from build123d import *

# Parameters (mm, degrees)
SKETCH1_R                = 6.5
SKETCH1_R_2              = 2
BOSS_EXTRUDE1_DEPTH      = 15
BOSS_EXTRUDE2_START      = -15
BOSS_EXTRUDE2_DEPTH      = 15
FILLET1_R                = 0.6
CIRPATTERN1_COUNT        = 10
FILLET1_OF_CIRPATTERN1_R = 0.6
BOSS_EXTRUDE3_START      = -15
BOSS_EXTRUDE3_DEPTH      = 15
BOSS_EXTRUDE4_DEPTH      = 7


with BuildPart() as part:
    # Sketch1 → Boss-Extrude1 (new body)
    with BuildSketch(Plane(origin=(0, 0, 0), x_dir=(1, 0, 0), z_dir=(0, 1, 0))):
        with Locations(Location((0, 0, 0), (0, 0, 270))):
            Circle(SKETCH1_R)
        with Locations(Location((0, 0, 0), (0, 0, 270))):
            Circle(SKETCH1_R_2, mode=Mode.SUBTRACT)
    extrude(amount=BOSS_EXTRUDE1_DEPTH)

    # Sketch2 → Boss-Extrude2 (add)
    with BuildSketch(Plane(origin=(0, 15, 0), x_dir=(1, 0, 0), z_dir=(0, 1, 0)).offset(BOSS_EXTRUDE2_START)):
        with BuildLine():
            Line((0.975354337, 8.443854802), (1.342832983, 6.359779837))
            ThreePointArc((1.342832983, 6.359779837), (0, 6.5), (-1.342832983, 6.359779837))
            Line((-1.342832983, 6.359779837), (-0.975354337, 8.443854802))
            ThreePointArc((-0.975354337, 8.443854802), (0, 8.5), (0.975354337, 8.443854802))
        make_face()
    boss_extrude2 = extrude(amount=BOSS_EXTRUDE2_DEPTH)

    # Fillet1
    fillet1_edges = [part.edges().sort_by_distance(p)[0] for p in [
        (-0.975354337, 7.5, -8.443854802),
        (0.975354337, 7.5, -8.443854802),
        (1.342832983, 7.5, -6.359779837),
        (-1.342832983, 7.5, -6.359779837),
    ]]
    fillet(fillet1_edges, radius=FILLET1_R)

    # CirPattern1: Boss-Extrude2 ×10 about axis
    cirpattern1_axis = Axis((0, 0, 0), (0, 1, 0))
    for i in range(1, CIRPATTERN1_COUNT):
        add(boss_extrude2.rotate(cirpattern1_axis, i * 360 / CIRPATTERN1_COUNT))

    # Fillet1 of CirPattern1
    fillet1_of_cirpattern1_edges = [part.edges().sort_by_distance(p)[0] for p in [
        (-5.752251559, 7.5, -6.257923138),
        (-4.174095091, 7.5, -7.404520928),
        (-2.651810092, 7.5, -5.934467393),
        (-4.8245595, 7.5, -4.355872545),
        (-8.331984198, 7.5, -1.681677534),
        (-7.729182066, 7.5, -3.53691173),
        (-5.633551844, 7.5, -3.242390109),
        (-6.463468269, 7.5, -0.688169991),
        (-7.729182066, 7.5, 3.53691173),
        (-8.331984198, 7.5, 1.681677534),
        (-6.463468269, 7.5, 0.688169991),
        (-5.633551844, 7.5, 3.242390109),
        (-4.174095091, 7.5, 7.404520928),
        (-5.752251559, 7.5, 6.257923138),
        (-4.8245595, 7.5, 4.355872545),
        (-2.651810092, 7.5, 5.934467393),
        (0.975354337, 7.5, 8.443854802),
        (-0.975354337, 7.5, 8.443854802),
        (-1.342832983, 7.5, 6.359779837),
        (1.342832983, 7.5, 6.359779837),
        (5.752251559, 7.5, 6.257923138),
        (4.174095091, 7.5, 7.404520928),
        (2.651810092, 7.5, 5.934467393),
        (4.8245595, 7.5, 4.355872545),
        (8.331984198, 7.5, 1.681677534),
        (7.729182066, 7.5, 3.53691173),
        (5.633551844, 7.5, 3.242390109),
        (6.463468269, 7.5, 0.688169991),
        (7.729182066, 7.5, -3.53691173),
        (8.331984198, 7.5, -1.681677534),
        (6.463468269, 7.5, -0.688169991),
        (5.633551844, 7.5, -3.242390109),
        (4.174095091, 7.5, -7.404520928),
        (5.752251559, 7.5, -6.257923138),
        (4.8245595, 7.5, -4.355872545),
        (2.651810092, 7.5, -5.934467393),
    ]]
    fillet(fillet1_of_cirpattern1_edges, radius=FILLET1_OF_CIRPATTERN1_R)

    # Sketch3 → Boss-Extrude3 (add)
    with BuildSketch(Plane(origin=(0, 15, 0), x_dir=(1, 0, 0), z_dir=(0, 1, 0)).offset(BOSS_EXTRUDE3_START)):
        with BuildLine():
            Line((-1.322875656, 1.5), (1.322875656, 1.5))
            ThreePointArc((1.322875656, 1.5), (0, 2), (-1.322875656, 1.5))
        make_face()
    extrude(amount=BOSS_EXTRUDE3_DEPTH)

    # Sketch4 → Boss-Extrude4 (add)
    with BuildSketch(Plane.XZ):
        with BuildLine():
            Line((1.322875656, -1.5), (-1.322875656, -1.5))
            ThreePointArc((-1.322875656, -1.5), (0, 2), (1.322875656, -1.5))
        make_face()
    extrude(amount=-BOSS_EXTRUDE4_DEPTH)


solid = part.part
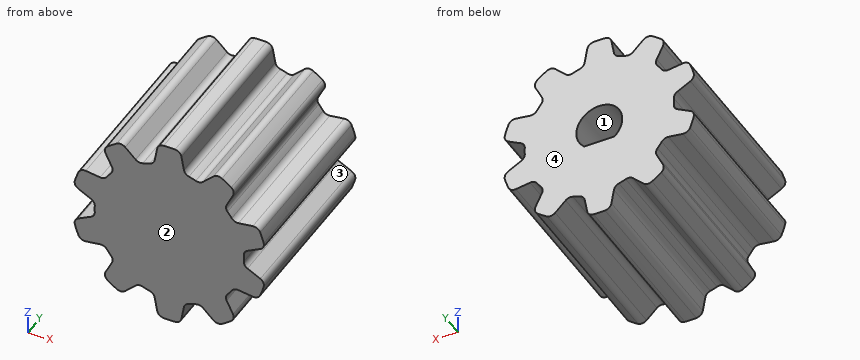
The model under review builds one solid part; all positions refer to its coordinate system, in mm. Face numbers are marked on the shaded views. A direction names the side the tool comes from. Give positions to 0.01 mm unless a question says otherwise; leave off trailing zeros. Order: outer loops, then holes, each group sorted by start corner. A loop starts at its lowest first (then second) coordinate and runs counter-clockwise, first axis right, second up. Notation, with made-up numbers: (-32, -21.75) -> (-13, -21.75) arc R21 cw to (-13, -10.75) -> close; hole circle Ø10 at (-28.5, 39). An arc over 180 degrees is marked (long way). Write item = value, one per line. Start each with the question number.
(1) Take a section at A-A (x = 0). Write out the cut boundary in (y, z), plus the area to 3 significant figures.
(2) Tool access review of the marked faces 3 and 4: name each direction out of +Z, -Z, +X, -X, +Y, -Y from which nothing blocks a thin tool from reaching the whole face with its end or side.
(3) Take a section at B-B (z = 0). Write out the cut boundary in (x, y).
(4) Draft analysis for pull direction Z (two halves, no side actions). For the marked faces 1 and 2, state which applies: +Z half, -Z half, draft (parallel to the pull), parting line (faces both ways), or undercut.
(5) Take a section at D-D (z = -5). Write out the cut boundary in (x, y), plus the area to 3 significant figures.
(6) For L1, parallel to Z at x = 0, y = 10.5; L2, parallel to Z at x = 5, y = 1.5; L3, parallel to X at y = 8.75, z = -7, list the stretches that pass through material, from the lowest coordinate up. Write a range as from..to.
(7) For pin 1 Ø6 at (x, y) = (-3.5, 3.5) entering from +Z; pin 2 Ø1 at (x, y) = (-4.5, 9.5) entering from +Z, all flat-tipped, find the tip position at first contact; note any pin that passes through.
(8) Take a section at C-C (x = 3.25). Write out the cut boundary in (y, z).
Returned:
q1.outline = (0, -8.5) -> (15, -8.5) -> (15, -1.5) -> (7, -1.5) -> (7, 2) -> (15, 2) -> (15, 8.5) -> (0, 8.5) -> close
q1.area = 227 mm²
q2.face_3 = +X, +Y, -Y
q2.face_4 = +Z, -Z, +X, -X, +Y
q3.outline = (-6.5, 0) -> (6.5, 0) -> (6.5, 15) -> (2, 15) -> (2, 7) -> (-2, 7) -> (-2, 15) -> (-6.5, 15) -> close
q4.face_1 = undercut
q4.face_2 = draft
q5.outline = (-5.14, 0) -> (5.14, 0) -> (5.14, 15) -> (-5.14, 15) -> close
q5.area = 154 mm²
q6.L1 = -8.5..-1.5, 2..8.5
q6.L2 = -6.87..-4.72, -4.18..4.18, 4.72..6.87
q6.L3 = -4.82..-3.76, -1.23..1.23, 3.76..4.82
q7.pin_1 = 8.49
q7.pin_2 = 7.25
q8.outline = (0, -6.51) -> (15, -6.51) -> (15, 6.51) -> (0, 6.51) -> close
